Read the model definition and answer for the solid it produces. Units are mm, in the model's axes. Face numbers are marked on the shaded views. A direction names the side the tool comes from. Give positions to 0.01 mm unless a question says otherwise; leave off trailing zeros. Write each loop counter-clockwise with the first axis right and the second up, starting at its lowest first coordinate (ties: lowest second). Pieces come first, ordered by that corner, then holes.
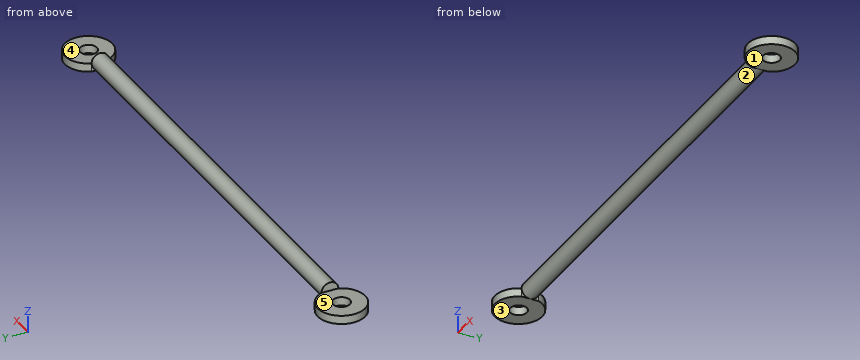
```python
from build123d import *

# Parameters (mm, degrees)
SKETCH1_W           = 131
SKETCH1_H           = 2.5
SKETCH3_R           = 2.5
BOSS_EXTRUDE2_DEPTH = 2.5


with BuildPart() as part:
    # Sketch1 → Revolve-Thin1 (revolve)
    with BuildSketch(Plane.XY):
        with Locations((0, 1.25)):
            Rectangle(SKETCH1_W, SKETCH1_H)
    revolve(axis=Axis((-65.5, 0, 0), (1, 0, 0)))

    # Sketch3 → Boss-Extrude2 (add)
    with BuildSketch(Plane.XY):
        with BuildLine():
            Line((65.5, 2.5), (65.5, -2.5))
            ThreePointArc((65.5, -2.5), (79.038348415, 0), (65.5, 2.5))
        make_face()
        with Locations((72.038348415, 0)):
            Circle(SKETCH3_R, mode=Mode.SUBTRACT)
        with BuildLine():
            Line((-65.5, -2.5), (-65.5, 2.5))
            ThreePointArc((-65.5, 2.5), (-79.038348415, 0), (-65.5, -2.5))
        make_face()
        with Locations((-72.038348415, 0)):
            Circle(SKETCH3_R, mode=Mode.SUBTRACT)
    extrude(amount=-BOSS_EXTRUDE2_DEPTH)


solid = part.part
```
Item 1: Section B-B (z = -1.4) is taken. Write down the section's boundary in (x, y), and give its area (3 significant figures).
Result set:
outline: (-65.5, -2.5) - (-65.5, -2.07) - (65.5, -2.07) - (65.5, -2.5) arc R7 ccw (long way) to (65.5, 2.5) - (65.5, 2.07) - (-65.5, 2.07) - (-65.5, 2.5) arc R7 ccw (long way) to start; hole circle Ø5 at (-72.04, 0); hole circle Ø5 at (72.04, 0)
area: 808 mm2
Item 2: Find the intervals of material crossed by line 1 along X through (y, z) = (2, -2.15); line 2 along X through (y, z) = (0.5, -0.65); line 3 along Z through (x, y) = (71, -5.75), in increasing order.
Result set:
line 1: x = -78.75 to -73.54, -70.54 to -65.5, 65.5 to 70.54, 73.54 to 78.75
line 2: x = -79.02 to -74.49, -69.59 to 69.59, 74.49 to 79.02
line 3: z = -2.5 to 0
Item 3: Determine the mould class of the marked faces 1 and 2 for opening direction X: pulls with the +X half, pulls with the -X half, needs draft (parallel to the pull), parting line crosses it, or undercut.
Result set:
face 1: needs draft
face 2: undercut
Item 4: Which of the six approach directions +Z, -Z, +X, -X, +Y, -Y give full straight-line access (tool end or side, diameter ignored) to the marked faces 3, 4 and 5?
Result set:
face 3: -Z, +X, -X, +Y, -Y
face 4: +Z, +X, +Y, -Y
face 5: +Z, -X, +Y, -Y
Item 5: Each of these flat-tipped pins is pushed along its axis until it touches: pin 1 Ø1.5 at (y, z) = (1, -2) entering from -X; pin 2 Ø2 at (y, z) = (-1, -1.5) entering from +X; pin 3 Ø3 at (x, y) = (2.5, 3) entering from -Z; pin 4 Ø6 at (x, y) = (-72.04, 0) entering from +Z. Where does it stop, or does it pass through?
Result set:
pin 1: stops at x = -79.03
pin 2: stops at x = 79.04
pin 3: stops at z = -2
pin 4: stops at z = 0
Item 6: Section A-A (y = -5.5) is taken. Write down the section's boundary in (x, z), and give its area (3 significant figures).
Result set:
outline: (-76.37, -2.5) - (-67.71, -2.5) - (-67.71, 0) - (-76.37, 0) - close; (67.71, -2.5) - (76.37, -2.5) - (76.37, 0) - (67.71, 0) - close
area: 43.3 mm2
Item 7: Section C-C (x = 1) is taken. Write down the section's boundary in (y, z), and give its area (3 significant figures).
Result set:
outline: circle Ø5 at (0, 0)
area: 19.6 mm2
